from build123d import *

# Parameters (mm, degrees)
EXTRUDE_1_DEPTH          = 13
SKETCH_3_R               = 31
CUT_EXTRUDE_1_DEPTH      = 3
CUT_EXTRUDE_3_DEPTH      = 53.630789468
CUT_EXTRUDE_3_DEPTH_BACK = 5
SKETCH_9_R               = 7
SKETCH_10_R              = 4.5
CUT_EXTRUDE_4_DEPTH      = 53.630789538


with BuildPart() as part:
    # Эскиз1 → Бобышка-Вытянуть1 (new, symmetric)
    with BuildSketch(Plane.XY):
        with BuildLine():
            Line((-28, 0), (-45, 0))
            Line((-45, 0), (-45, -24))
            Line((-45, -24), (-40.657102701, -24))
            ThreePointArc((-40.657102701, -24), (-36.423365781, -24.940448593), (-32.985951248, -27.58490566))
            ThreePointArc((-32.985951248, -27.58490566), (0, -43), (32.985951248, -27.58490566))
            ThreePointArc((32.985951248, -27.58490566), (36.423365781, -24.940448593), (40.657102701, -24))
            Line((40.657102701, -24), (45, -24))
            Line((45, -24), (45, 0))
            Line((45, 0), (28, 0))
            ThreePointArc((28, 0), (0, -28), (-28, 0))
        make_face()
    extrude(amount=EXTRUDE_1_DEPTH, both=True)

    # Эскиз3 → Вырез-Вытянуть1 (cut)
    with BuildSketch(Plane.XY.offset(-13)):
        Circle(SKETCH_3_R)
    cut_extrude_1 = extrude(amount=CUT_EXTRUDE_1_DEPTH, mode=Mode.SUBTRACT)

    # Зеркальное отражение2: Вырез-Вытянуть1 across plane
    add(cut_extrude_1.mirror(Plane.XY), mode=Mode.SUBTRACT)

    # Эскиз9 → Вырез-Вытянуть3 (cut, two sides: drawn at the far end of the back side and taken through both)
    with BuildSketch(Plane.XZ.offset(24).offset(-CUT_EXTRUDE_3_DEPTH_BACK)):
        with Locations((-37, 0)):
            Circle(SKETCH_9_R)
        with Locations((37, 0)):
            Circle(SKETCH_9_R)
    extrude(amount=CUT_EXTRUDE_3_DEPTH + CUT_EXTRUDE_3_DEPTH_BACK, mode=Mode.SUBTRACT)

    # Эскиз10 → Вырез-Вытянуть4 (cut, through all)
    with BuildSketch(Plane.XZ.offset(19)):
        with Locations((-37, 0)):
            Circle(SKETCH_10_R)
        with Locations((37, 0)):
            Circle(SKETCH_10_R)
    extrude(amount=-CUT_EXTRUDE_4_DEPTH, mode=Mode.SUBTRACT)


solid = part.part
CAD build for the part. Positions are in the model's coordinates, mm. A direction names the side the tool comes from. Coordinates: 2 decimals unless noted, no trailing zeros. Loops run counter-clockwise (first coordinate to the right, second up) from the corner with the lowest first, then second, coordinate; pieces in that order, holes last. Notation, with made-up numbers: (2.5, 72) -> (38.5, 72) arc R28 cw to (38.5, 91) -> close; hole circle Ø11 at (0.5, 29.5). An arc over 180 degrees is marked (long way). One line per item, written item: value.
1. Slice it at A-A on y = -8.5. Write the cut outline in (x, z), and give its area (3 significant figures).
Answers:
outline: (-45, -13) -> (-29.81, -13) -> (-29.81, -10) -> (-26.68, -10) -> (-26.68, 10) -> (-29.81, 10) -> (-29.81, 13) -> (-45, 13) -> close; (26.68, -10) -> (29.81, -10) -> (29.81, -13) -> (45, -13) -> (45, 13) -> (29.81, 13) -> (29.81, 10) -> (26.68, 10) -> close; hole circle Ø9 at (-37, 0); hole circle Ø9 at (37, 0)
area: 788 mm^2
2. Slice it at B-B on z = -2.25. Write the cut outline in (x, y), and give its area (3 significant figures).
Answers:
outline: (-45, -24) -> (-43.63, -24) -> (-43.63, -19) -> (-40.9, -19) -> (-40.9, 0) -> (-45, 0) -> close; (-33.1, -19) -> (-30.37, -19) -> (-30.37, -30.44) arc R43 ccw to (30.37, -30.44) -> (30.37, -19) -> (33.1, -19) -> (33.1, 0) -> (28, 0) arc R28 cw to (-28, 0) -> (-33.1, 0) -> close; (40.9, -19) -> (43.63, -19) -> (43.63, -24) -> (45, -24) -> (45, 0) -> (40.9, 0) -> close
area: 1,420 mm^2
3. Pull direction X, two halves, no side cores. Call faces 6 (the face through (-30.323, -23.509, 2.103)), 7 (the face through (-0.526, -42.997, 0.182)), 8 (the face through (-36.479, -24.915, -10.124)), 9 (the face through (33, 0, 3)): pulls with the +X half, pulls with the -X half, needs draft (parallel to the pull), parting line crosses it, or undercut.
Answers:
face 6: undercut
face 7: parting line crosses it
face 8: pulls with the -X half
face 9: needs draft
4. Drill centre lines: line 1 (X direction, y = -6, z = -3.25); line 2 (Z direction, x = 37, y = -24.25); line 3 (Z direction, x = -37, y = -7). Where is each one in solid material? Low to high. Write a range as [from, to].
Answers:
line 1: x = [-45, -40.11], [-33.89, -27.35], [27.35, 33.89], [40.11, 45]
line 2: z = [-13, -7], [7, 13]
line 3: z = [-13, -4.5], [4.5, 13]
5. Slice it at C-C on x = 0. Write the cut outline in (y, z), and give its area (3 significant figures).
Answers:
outline: (-43, -13) -> (-31, -13) -> (-31, -10) -> (-28, -10) -> (-28, 10) -> (-31, 10) -> (-31, 13) -> (-43, 13) -> close
area: 372 mm^2
6. Flat gauge pins, fed straight in: P1, Ø4, axis at x = 0, z = 0.5, coming from the +Y side; P2, Ø5, axis at x = 42, z = -1, coming from the -Y side; P3, Ø4, axis at x = 34, z = 2.5, coming from the -Y side; P4, Ø8, axis at x = -37, z = 0, coming from the +Y side. Where does each tip first touch, or does it go through?
Answers:
P1: stops at y = -27.93
P2: stops at y = -24
P3: stops at y = -19
P4: passes through
7. Which spindle directions (+Z, -Z, +X, -X, +Y, -Y) get a long thin tool onto all of the face, cutting with end or side? Do faces 1 (the face through (44.2, -24, 0.2)), 2 (the face through (37, -19, -5)), 3 (the face through (-44.3, -24, 0.2)), 4 (the face through (-0.682, -30.993, 11.521)), 5 (the face through (-0.682, -30.993, -11.521)). Say none if no direction does.
Answers:
face 1: +Z, -Z, +X, -Y
face 2: -Y
face 3: +Z, -Z, -X, -Y
face 4: +Z, +Y
face 5: -Z, +Y
8. Slice it at D-D on x = -37. Write the cut outline in (y, z).
Answers:
outline: (-24.69, -13) -> (0, -13) -> (0, -4.5) -> (-19, -4.5) -> (-19, -7) -> (-24.69, -7) -> close; (-24.69, 7) -> (-19, 7) -> (-19, 4.5) -> (0, 4.5) -> (0, 13) -> (-24.69, 13) -> close
